from build123d import *

# Parameters (mm, degrees)
SKETCH1_R           = 1.5
BOSS_EXTRUDE1_DEPTH = 3
FILLET5_RADIUS      = 10
FILLET5_LENGTH      = 3
FILLET2_R           = 5.4
FILLET4_R           = 5.4


with BuildPart() as part:
    # Sketch1 → Boss-Extrude1 (new body)
    # profile 1 of 2: a face of its own
    with BuildSketch(Plane(origin=(0, 0, 0), x_dir=(1, 0, 0), z_dir=(0, 1, 0))):
        with BuildLine():
            Line((3.5, 25), (0, 25))
            Line((0, 25), (0, 15))
            Line((0, 15), (10, 0))
            Line((10, 0), (26, 0))
            Line((26, 0), (36, 15))
            Line((36, 15), (60, 15))
            Line((60, 15), (60, 25))
            Line((60, 25), (44.5, 25))
            Line((44.5, 25), (44.5, 19.6))
            Line((44.5, 19.6), (26.5, 19.6))
            Line((26.5, 19.6), (26.5, 25))
            Line((26.5, 25), (6.5, 25))
            ThreePointArc((6.5, 25), (5, 23.5), (3.5, 25))
        make_face()
        with Locations(Location((13, 5, 0), (0, 0, 270))):
            Circle(SKETCH1_R, mode=Mode.SUBTRACT)
        with Locations(Location((23, 5, 0), (0, 0, 270))):
            Circle(SKETCH1_R, mode=Mode.SUBTRACT)
    # profile 2 of 2: a face of its own
    with BuildSketch(Plane(origin=(0, 0, 0), x_dir=(1, 0, 0), z_dir=(0, 1, 0))):
        with BuildLine():
            Line((10, 45), (0, 33.819660113))
            Line((0, 33.819660113), (0, 25))
            Line((0, 25), (3.5, 25))
            ThreePointArc((3.5, 25), (5, 26.5), (6.5, 25))
            Line((6.5, 25), (26.5, 25))
            Line((26.5, 25), (26.5, 30.4))
            Line((26.5, 30.4), (44.5, 30.4))
            Line((44.5, 30.4), (44.5, 25))
            Line((44.5, 25), (60, 25))
            Line((60, 25), (60, 35))
            Line((60, 35), (36, 35))
            Line((36, 35), (26, 45))
            Line((26, 45), (10, 45))
        make_face()
    extrude(amount=BOSS_EXTRUDE1_DEPTH)

    # Fillet5: full round fillet: the end face becomes a half cylinder, R = half its width
    fillet5_face = Plane((60, 1.5, -25), x_dir=(0, -1, 0), z_dir=(1, 0, 0))  # on the end face: x along it, z out of the body
    fillet5_slab = fillet5_face.offset(-FILLET5_RADIUS / 2) * Box(FILLET5_LENGTH, 2 * FILLET5_RADIUS, FILLET5_RADIUS, mode=Mode.PRIVATE)  # the body's end, R deep
    fillet5_round = Plane((50, 1.5, -25), x_dir=(1, 0, 0), z_dir=(0, -1, 0)) * Cylinder(FILLET5_RADIUS, FILLET5_LENGTH, mode=Mode.PRIVATE)  # its axis R under the face
    add(fillet5_slab - fillet5_round, mode=Mode.SUBTRACT)

    # Fillet2
    fillet2_edges = [part.edges().sort_by_distance(p)[0] for p in [
        (26.5, 1.5, -30.4),
        (26.5, 1.5, -19.6),
    ]]
    fillet(fillet2_edges, radius=FILLET2_R - 0.0001)  # a hair under: the kernel refuses the full size

    # Fillet4
    fillet4_edges = [part.edges().sort_by_distance(p)[0] for p in [
        (44.5, 1.5, -19.6),
        (44.5, 1.5, -30.4),
    ]]
    fillet(fillet4_edges, radius=FILLET4_R - 0.0001)  # a hair under: the kernel refuses the full size


solid = part.part
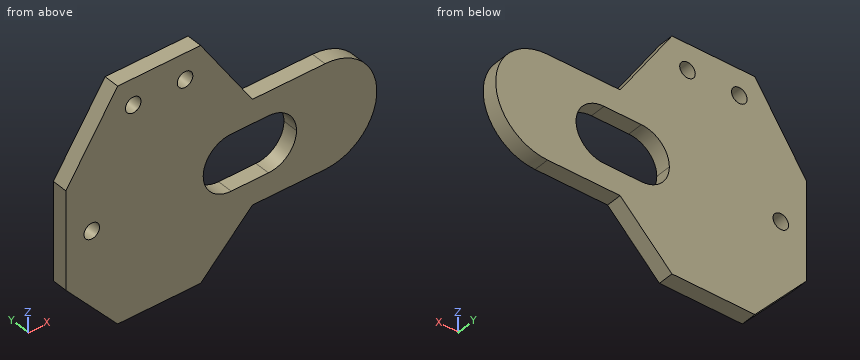
Geometry check sheet. Reference: the model listing, model coordinates, mm. Give positions to 0.01 mm unless a question says otherwise; leave off trailing zeros. Write each loop counter-clockwise with the first axis right and the second up, starting at its lowest first coordinate (ties: lowest second). Pieces come first, ordered by that corner, then holes.
1) Cross-section at A-A (y = 0.45). Count the separate pieces of the cut face and the enclosed holes in it, plus the area to 3 significant figures.
Values follow:
separate pieces: 1
enclosed holes: 4
area: 1,610 mm2
2) Go/stop test with flat-tipped pins: pin 1 Ø0.9 at (x, y) = (36.5, 1.5) entering from -Z; pin 2 Ø12 at (x, z) = (38.5, -32) entering from -Y; pin 3 Ø1.5 at (y, z) = (1, -27) entering from +X. Record where each tip stops, or that it passes through.
Values follow:
pin 1: stops at z = -35
pin 2: stops at y = 0
pin 3: stops at x = 59.92
3) Cross-section at D-D (z = -27.5). Record the boundary of the cut face in (x, y).
Values follow:
outline: (0, 0) - (27.11, 0) - (27.11, 3) - (0, 3) - close; (43.89, 0) - (59.68, 0) - (59.68, 3) - (43.89, 3) - close
4) Cross-section at C-C (z = -5). Record the boundary of the cut face in (x, y), plus the area to 3 significant figures.
Values follow:
outline: (6.67, 0) - (11.5, 0) - (11.5, 3) - (6.67, 3) - close; (14.5, 0) - (21.5, 0) - (21.5, 3) - (14.5, 3) - close; (24.5, 0) - (29.33, 0) - (29.33, 3) - (24.5, 3) - close
area: 50.0 mm2
5) Thickness scan on line 1 (X direction, y = 1.7, z = -25); line 2 (Z direction, x = 36.5, y = 2.8); line 3 (X direction, y = 1.45, z = -5). Record the ranges inside material, lowest first.
Values follow:
line 1: x = 0 to 3.5, 6.5 to 26.5, 44.5 to 60
line 2: z = -35 to -30.4, -19.6 to -15
line 3: x = 6.67 to 11.5, 14.5 to 21.5, 24.5 to 29.33
6) Cross-section at B-B (x = 5). Record the boundary of the cut face in (y, z), plus the area to 3 significant figures.
Values follow:
outline: (0, -39.41) - (3, -39.41) - (3, -26.5) - (0, -26.5) - close; (0, -23.5) - (3, -23.5) - (3, -7.5) - (0, -7.5) - close
area: 86.7 mm2
